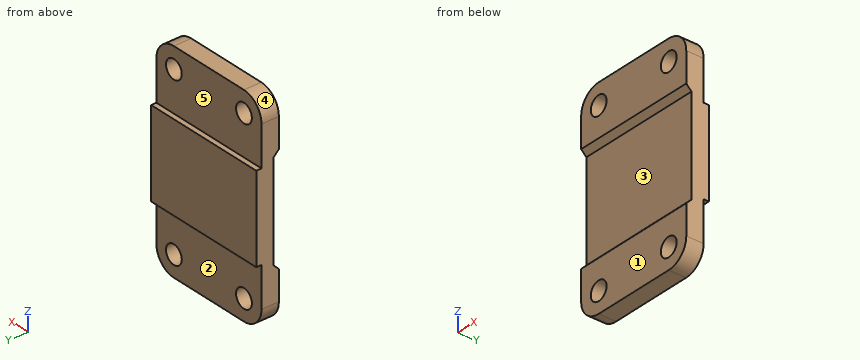
from build123d import *

# Parameters (mm, degrees)
BOSS_EXTRUDE1_DEPTH     = 36
FILLET1_R               = 12
M12X1_25_TAPPED_HOLE1_D = 10.8


with BuildPart() as part:
    # Sketch1 → Boss-Extrude1 (new, symmetric)
    with BuildSketch(Plane(origin=(0, 0, 0), x_dir=(0, 0, -1), z_dir=(1, 0, 0))):
        Polygon((-28, 3), (-31, 0), (-60, 0), (-60, 10), (-25, 10), (-25, 13), (25, 13), (25, 10), (60, 10), (60, 0), (31, 0), (28, 3), align=None)
    extrude(amount=BOSS_EXTRUDE1_DEPTH, both=True)

    # Fillet1
    fillet1_edges = [part.edges().sort_by_distance(p)[0] for p in [
        (-36, 5, 60),
        (-36, 5, -60),
        (36, 5, -60),
        (36, 5, 60),
    ]]
    fillet(fillet1_edges, radius=FILLET1_R)

    # M12x1.25 Tapped Hole1 (through all)
    with Locations(Plane(origin=(0, 10, 0), x_dir=(1, 0, 0), z_dir=(0, 1, 0))):
        with Locations((24, -48), (-24, -48), (24, 48), (-24, 48)):
            Hole(M12X1_25_TAPPED_HOLE1_D / 2)


solid = part.part
CAD build for the part. Positions are in the model's coordinates, mm. Face numbers are marked on the shaded views. A direction names the side the tool comes from. Give positions to 0.01 mm unless a question says otherwise; leave off trailing zeros. Write each loop counter-clockwise with the first axis right and the second up, starting at its lowest first coordinate (ties: lowest second). Pieces come first, ordered by that corner, then holes. Notation, with made-up numbers: (23, -19.5) - (59, -19.5) arc R31 cw to (59, 5.5) - close; hole circle Ø8 at (85.25, -19). An arc over 180 degrees is marked (long way). Answer as CSV lines item,"result".
Q1. Pull direction Z, two halves, no side cores. Call the marked faces 3, 4 and 5: released by +Z, released by -Z, zero draft, split by the parting line, or undercut.
Result set:
face 3,"undercut"
face 4,"released by +Z"
face 5,"zero draft"
Q2. Band-saw the part on C-C (x = -22). Give the cut face in (y, z).
Result set:
outline,"(0, -60) - (10, -60) - (10, -53.02) - (0, -53.02) - close; (0, -42.98) - (10, -42.98) - (10, -25) - (13, -25) - (13, 25) - (10, 25) - (10, 42.98) - (0, 42.98) - (0, 31) - (3, 28) - (3, -28) - (0, -31) - close; (0, 53.02) - (10, 53.02) - (10, 60) - (0, 60) - close"
Q3. 3-axis set-ups, long thin cutter, end or side, ignore diameter. For the marked faces 1 and 2: which of +Z, -Z, +X, -X, +Y, -Y reach the whole face in a straight line?
Result set:
face 1,"+Z, -Z, +X, -X, -Y"
face 2,"-Z, +X, -X, +Y"
Q4. Flat gauge pins, fed straight in: pin 1 Ø3.5 at (x, y) = (11.5, 11.5) entering from -Z; pin 2 Ø8.5 at (x, z) = (-24, 48) entering from +Y; pin 3 Ø17.5 at (x, z) = (24, -48) entering from +Y; pin 4 Ø6 at (x, z) = (9, 6) entering from -Y. Where does each tip first touch, or does it go through?
Result set:
pin 1,"z = -60"
pin 2,"through"
pin 3,"y = 10"
pin 4,"y = 3"
Q5. Band-saw the part on B-B (z = -45.5). Give the cut face in (x, y).
Result set:
outline,"(-36, 0) - (-28.79, 0) - (-28.79, 10) - (-36, 10) - close; (-19.21, 0) - (19.21, 0) - (19.21, 10) - (-19.21, 10) - close; (28.79, 0) - (36, 0) - (36, 10) - (28.79, 10) - close"
Q6. Drill centre lines: line 1 (Z direction, x = 24, y = 7.75); line 2 (X direction, y = 6.5, z = -48); line 3 (X direction, y = 1.75, z = -43). Where is each one in solid material? Low to high. Write a range as from..to.
Result set:
line 1,"-60..-53.4, -42.6..42.6, 53.4..60"
line 2,"-36..-29.4, -18.6..18.6, 29.4..36"
line 3,"-36..-26.04, -21.96..21.96, 26.04..36"
Q7. Band-saw the part on A-A (y = 8). Give the cut face in (x, z), and give its area (3 significant figures).
Result set:
outline,"(-36, -48) arc R12 ccw to (-24, -60) - (24, -60) arc R12 ccw to (36, -48) - (36, 48) arc R12 ccw to (24, 60) - (-24, 60) arc R12 ccw to (-36, 48) - close; hole circle Ø10.8 at (-24, -48); hole circle Ø10.8 at (-24, 48); hole circle Ø10.8 at (24, -48); hole circle Ø10.8 at (24, 48)"
area,"8,150 mm²"
Q8. Band-saw the part on D-D (x = 15). Give the cut face in (y, z), and give its area (3 significant figures).
Result set:
outline,"(0, -60) - (10, -60) - (10, -25) - (13, -25) - (13, 25) - (10, 25) - (10, 60) - (0, 60) - (0, 31) - (3, 28) - (3, -28) - (0, -31) - close"
area,"1,170 mm²"
